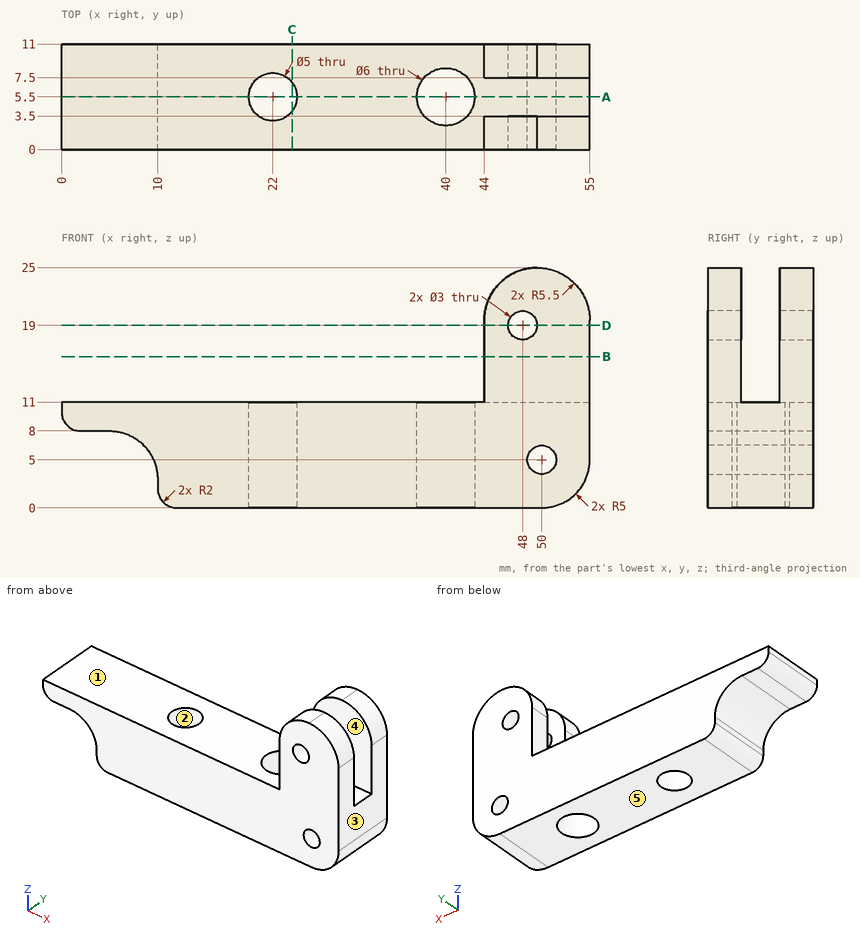
Could you check a few things on this drawing? It's one solid part, dimensions in mm from its lowest x, y, z. A direction names the side the tool comes from. Coordinates: 2 decimals unless noted, no trailing zeros. Write each loop counter-clockwise with the first axis right and the second up, starting at its lowest first coordinate (ties: lowest second). Pieces come first, ordered by that corner, then holes.
Q1. Imagine slicing it at C-C, the plane x = 24. List the corners of the cut face in (y, z) for me, plus the area to 3 significant figures.
Results found:
outline: (0, 0) - (4, 0) - (4, 11) - (0, 11) - close; (7, 0) - (11, 0) - (11, 11) - (7, 11) - close
area: 88.0 mm2
Q2. Imagine slicing it at D-D, the plane z = 19. List the corners of the cut face in (x, y) for me.
Results found:
outline: (44, 0) - (46.5, 0) - (46.5, 3.5) - (44, 3.5) - close; (44, 7.5) - (46.5, 7.5) - (46.5, 11) - (44, 11) - close; (49.5, 0) - (55, 0) - (55, 3.5) - (49.5, 3.5) - close; (49.5, 7.5) - (55, 7.5) - (55, 11) - (49.5, 11) - close
Q3. Imagine slicing it at B-B, the plane z = 15.75. List the corners of the cut face in (x, y) for me, plus the area to 3 significant figures.
Results found:
outline: (44, 0) - (55, 0) - (55, 3.5) - (44, 3.5) - close; (44, 7.5) - (55, 7.5) - (55, 11) - (44, 11) - close
area: 77.0 mm2
Q4. Please list where these lines run through material, in increasing order: L1, parallel to X at y = 8.65, z = 19; L2, parallel to Y at x = 22, z = 6.5; L3, parallel to Y at x = 40, z = 4.25.
Results found:
L1: x = 44 to 46.5, 49.5 to 55
L2: y = 0 to 3, 8 to 11
L3: y = 0 to 2.5, 8.5 to 11
Q5. If we mould it in two halves opening along X, with no side actions, what happens to the marked faces 1, 2 and 3? For each: +X half, -X half, draft (parallel to the pull), parting line (faces both ways), or undercut.
Results found:
face 1: draft
face 2: undercut
face 3: +X half
Q6. Which directions (+Z, -Z, +X, -X, +Y, -Y) give clear straight access to the entire face, cutting with the end or side of a thin tool? Please do the marked faces 4 and 5.
Results found:
face 4: +Z, +X, -X
face 5: -Z, +X, -X, +Y, -Y
Q7. For P1, Ø5.5, axis at x = 52, z = 16, coming from the -Y side; P2, Ø0.5, axis at y = 7, z = 2.5, coming from the -X side; P3, Ø3.5, axis at x = 4, y = 8, coming from the -Z side; P4, Ø2.5, axis at x = 48, z = 19, coming from the -Y side, each with a flat end and sliding along its axis, tell me the tip position at first contact or that it passes through.
Results found:
P1: stops at y = 0
P2: stops at x = 10
P3: stops at z = 7.94
P4: passes through
Q8. Imagine slicing it at A-A, the plane y = 5.5. List the corners of the cut face in (x, z) for me.
Results found:
outline: (0, 10) arc R2 ccw to (2, 8) - (5, 8) arc R5 cw to (10, 3) - (10, 2) arc R2 ccw to (12, 0) - (19.5, 0) - (19.5, 11) - (0, 11) - close; (24.5, 0) - (37, 0) - (37, 11) - (24.5, 11) - close; (43, 0) - (50, 0) arc R5 ccw to (55, 5) - (55, 11) - (43, 11) - close; hole circle Ø3 at (50, 5)
